Read the model definition and answer for the solid it produces. Units are mm, in the model's axes. A direction names the side the tool comes from. Coordinates: 2 decimals unless noted, no trailing zeros. Order: outer loops, then holes, each group sorted by start corner. A loop starts at its lowest first (then second) coordinate and runs counter-clockwise, first axis right, second up. Notation, with made-up numbers: M 22.5,85 L 71.5,85 A27 cw 71.5,105 Z; hole C 11.25,52 d6. An arc over 180 degrees is marked long. Use a Markdown table: item, result. Add a question column.
1) Each of these flat-tipped pins is pushed along its axis until it touches: pin 1 Ø2 at (x, y) = (45.5, -19) entering from -Z; pin 2 Ø8 at (y, z) = (-32, 12) entering from +X; pin 3 Ø5.5 at (x, y) = (402.5, -28) entering from -Z; pin 4 Ø10 at (x, z) = (143.5, 24) entering from +Y. Where does it stop, or does it pass through?
2) For faces 5 (the face through (395, -25, 11.195)), 6 (the face through (200, -29, 19.35)), 7 (the face through (431, -34, 12)), determine the directions among +Z, -Z, +X, -X, +Y, -Y from which every point of the face is accessible in a straight line to the end or side of a thin tool.
3) The mould has two halves that part along X. Classify faces 1 (the face through (385, -25, 6)), 2 (the face through (498, -10, 17)), 3 (the face through (75, -25, 0)), 4 (the face through (87, -31, 13)): released by +X, released by -X, zero draft, split by the parting line, or undercut.
4) Find the intervals of material crossed by probe 1 along Y at (x, z) = (402.5, 20.25); probe 2 along X at (y, z) = (-15.5, 8.5); probe 3 along X at (y, z) = (-21, 22), in increasing order. Write a range as [from, to].
5) Find section A-A on x = 194. Write down the section's boundary in (y, z).
from build123d import *

# Parameters (mm, degrees)
SKETCH6_R             = 9
BOSS_EXTRUDE2_DEPTH   = 27
CHAMFER1_SIZE         = 4
CUT_EXTRUDE5_DEPTH    = 28
CHAMFER2_SIZE         = 0.5
CHAMFER3_SIZE         = 0.5
SKETCH8_W             = 30
SKETCH8_H             = 16
CUT_EXTRUDE6_DEPTH    = 27
SKETCH8_3_W           = 30
SKETCH8_3_H           = 27
CUT_EXTRUDE7_DEPTH    = 4
FILLET1_R             = 2
CUT_EXTRUDE8_DEPTH    = 1
SKETCH11_W            = 21
SKETCH11_H            = 28.648086621
CUT_EXTRUDE9_DEPTH    = 51
SKETCH12_W            = 21
SKETCH12_H            = 8
CUT_EXTRUDE10_DEPTH   = 20
SKETCH13_W            = 21
SKETCH13_H            = 30.21821637
CUT_EXTRUDE11_DEPTH   = 51
CUT_EXTRUDE12_DEPTH   = 34.38478555
SKETCH15_R            = 1.75
CUT_EXTRUDE13_DEPTH   = 28
SKETCH16_R            = 3.25
CUT_EXTRUDE14_DEPTH   = 3.5
FILLET2_R             = 1
M4_TAPPED_HOLE1_D     = 3.3
M4_TAPPED_HOLE1_DEPTH = 8
M4_TAPPED_HOLE1_TIP   = 0.991420021
M3_TAPPED_HOLE1_D     = 2.5
M3_TAPPED_HOLE1_DEPTH = 6
M3_TAPPED_HOLE1_TIP   = 0.751075774
M3_TAPPED_HOLE2_D     = 2.5
M3_TAPPED_HOLE2_DEPTH = 6
M3_TAPPED_HOLE2_TIP   = 0.751075774
M3_TAPPED_HOLE3_D     = 2.5
M3_TAPPED_HOLE3_DEPTH = 6
M3_TAPPED_HOLE3_TIP   = 0.751075774
M3_TAPPED_HOLE4_D     = 2.5
M3_TAPPED_HOLE4_DEPTH = 6
M3_TAPPED_HOLE4_TIP   = 0.751075774
M3_TAPPED_HOLE5_D     = 2.5
M3_TAPPED_HOLE5_DEPTH = 6
M3_TAPPED_HOLE5_TIP   = 0.751075774
SKETCH29_W            = 25.5
SKETCH29_H            = 8
CUT_EXTRUDE15_DEPTH   = 17.61521445


with BuildPart() as part:
    # Sketch6 → Boss-Extrude2 (new body)
    with BuildSketch(Plane.XY):
        Polygon((112, -50), (477, -50), (477, -19), (498, -19), (498, 0), (214.9, 0), (214.9, -16.61521445), (137.1, -16.61521445), (137.1, 0), (0, 0), (0, -50), (87, -50), (87, -16.61521445), (112, -16.61521445), align=None)
        with Locations((27, -37)):
            Circle(SKETCH6_R, mode=Mode.SUBTRACT)
        with Locations((461, -37)):
            Circle(SKETCH6_R, mode=Mode.SUBTRACT)
    extrude(amount=BOSS_EXTRUDE2_DEPTH)

    # Chamfer1
    chamfer1_edges = [part.edges().sort_by_distance(p)[0] for p in [
        (0, -50, 13.5),
    ]]
    chamfer(chamfer1_edges, length=CHAMFER1_SIZE)

    # Sketch7 → Cut-Extrude5 (cut, through all)
    with BuildSketch(Plane.XY.offset(27)):
        with BuildLine():
            Line((151, -41.853199992), (151, -50))
            Line((151, -50), (165, -50))
            Line((165, -50), (165, -41.853199992))
            ThreePointArc((165, -41.853199992), (158, -34.853199992), (151, -41.853199992))
        make_face()
        with BuildLine():
            Line((187, -50), (201, -50))
            Line((201, -50), (201, -41.853199992))
            ThreePointArc((201, -41.853199992), (194, -34.853199992), (187, -41.853199992))
            Line((187, -41.853199992), (187, -50))
        make_face()
    extrude(amount=-CUT_EXTRUDE5_DEPTH, mode=Mode.SUBTRACT)

    # Chamfer2
    chamfer2_edges = [part.edges().sort_by_distance(p)[0] for p in [
        (137.1, 0, 13.5),
        (214.9, 0, 13.5),
    ]]
    chamfer(chamfer2_edges, length=CHAMFER2_SIZE)

    # Chamfer3
    chamfer3_edges = [part.edges().sort_by_distance(p)[0] for p in [
        (0, 0, 13.5),
        (498, 0, 13.5),
        (477, -50, 13.5),
        (112, -50, 13.5),
        (87, -50, 13.5),
    ]]
    chamfer(chamfer3_edges, length=CHAMFER3_SIZE)

    # Sketch8 → Cut-Extrude6 (cut)
    with BuildSketch(Plane.XY.offset(27)):
        with Locations((431, -42)):
            Rectangle(SKETCH8_W, SKETCH8_H)
    extrude(amount=-CUT_EXTRUDE6_DEPTH, mode=Mode.SUBTRACT)

    # Sketch8<3> → Cut-Extrude7 (cut)
    with BuildSketch(Plane.XY.offset(27)):
        with Locations((431, -20.5)):
            Rectangle(SKETCH8_3_W, SKETCH8_3_H)
    extrude(amount=-CUT_EXTRUDE7_DEPTH, mode=Mode.SUBTRACT)

    # Fillet1
    fillet1_edges = [part.edges().sort_by_distance(p)[0] for p in [
        (416, -7, 25),
        (446, -7, 25),
    ]]
    fillet(fillet1_edges, radius=FILLET1_R)

    # Sketch10 → Cut-Extrude8 (cut)
    with BuildSketch(Plane.XY.offset(27)):
        Polygon((5, -4.129705764), (132.1, -4.129705764), (137.1, -5.469451726), (137.1, -4.129705764), (493, -4.129705764), (498, -5.469451726), (498.112682479, -4.129705764), (498.112682479, 0), (0, 0), (0, -4.129705764), (0, -5.469451726), align=None)
    extrude(amount=-CUT_EXTRUDE8_DEPTH, mode=Mode.SUBTRACT)

    # Sketch11 → Cut-Extrude9 (cut, through all)
    with BuildSketch(Plane.XZ.offset(50)):
        with Locations((53.5, -6.324043311)):
            Rectangle(SKETCH11_W, SKETCH11_H)
    extrude(amount=-CUT_EXTRUDE9_DEPTH, mode=Mode.SUBTRACT)

    # Sketch12 → Cut-Extrude10 (cut, through all)
    with BuildSketch(Plane.XZ.offset(19)):
        with Locations((487.5, 4)):
            Rectangle(SKETCH12_W, SKETCH12_H)
    extrude(amount=-CUT_EXTRUDE10_DEPTH, mode=Mode.SUBTRACT)

    # Sketch13 → Cut-Extrude11 (cut, through all)
    with BuildSketch(Plane.XZ.offset(50)):
        with Locations((395.5, -3.9138874)):
            Rectangle(SKETCH13_W, SKETCH13_H)
    extrude(amount=-CUT_EXTRUDE11_DEPTH, mode=Mode.SUBTRACT)

    # Sketch14 → Cut-Extrude12 (cut, through all)
    with BuildSketch(Plane(origin=(0, -16.61521445, 0), x_dir=(1, 0, 0), z_dir=(0, 1, 0))):
        Polygon((137.1, -27), (214.9, -27), (214.9, -19.35), (184, -19.35), (184, -16.3), (167.5, -16.3), (167.5, -19.35), (137.1, -19.35), align=None)
    extrude(amount=-CUT_EXTRUDE12_DEPTH, mode=Mode.SUBTRACT)

    # Sketch15 → Cut-Extrude13 (cut, through all)
    with BuildSketch(Plane.XY.offset(27)):
        with Locations((45.5, -19)):
            Circle(SKETCH15_R)
        with Locations((60.5, -19)):
            Circle(SKETCH15_R)
        with Locations((45.5, -28)):
            Circle(SKETCH15_R)
        with Locations((60.5, -28)):
            Circle(SKETCH15_R)
        with Locations((387.5, -19)):
            Circle(SKETCH15_R)
        with Locations((402.5, -19)):
            Circle(SKETCH15_R)
        with Locations((387.5, -28)):
            Circle(SKETCH15_R)
        with Locations((402.5, -28)):
            Circle(SKETCH15_R)
    extrude(amount=-CUT_EXTRUDE13_DEPTH, mode=Mode.SUBTRACT)

    # Sketch16 → Cut-Extrude14 (cut)
    with BuildSketch(Plane.XY.offset(27)):
        with Locations((45.5, -19)):
            Circle(SKETCH16_R)
        with Locations((60.5, -19)):
            Circle(SKETCH16_R)
        with Locations((60.5, -28)):
            Circle(SKETCH16_R)
        with Locations((45.5, -28)):
            Circle(SKETCH16_R)
        with Locations((387.5, -19)):
            Circle(SKETCH16_R)
        with Locations((402.5, -19)):
            Circle(SKETCH16_R)
        with Locations((402.5, -28)):
            Circle(SKETCH16_R)
        with Locations((387.5, -28)):
            Circle(SKETCH16_R)
    extrude(amount=-CUT_EXTRUDE14_DEPTH, mode=Mode.SUBTRACT)

    # Fillet2
    fillet2_edges = [part.edges().sort_by_distance(p)[0] for p in [
        (137.1, -16.61521445, 9.675),
        (214.9, -16.61521445, 9.675),
    ]]
    fillet(fillet2_edges, radius=FILLET2_R)

    # M4 Tapped Hole1
    with Locations(Plane.XY.offset(19.35)):
        with Locations((146, -27), (206, -27)):
            Hole(M4_TAPPED_HOLE1_D / 2, depth=M4_TAPPED_HOLE1_DEPTH)
            with Locations((0, 0, -(M4_TAPPED_HOLE1_DEPTH + M4_TAPPED_HOLE1_TIP / 2))):  # 118° drill point
                Cone(0, M4_TAPPED_HOLE1_D / 2, M4_TAPPED_HOLE1_TIP, mode=Mode.SUBTRACT)

    # M3 Tapped Hole1
    with Locations(Plane.XY.offset(27)):
        with Locations((13, -10), (33, -10), (80, -10), (110, -10), (251, -10), (303, -10), (373, -10), (358, -10)):
            Hole(M3_TAPPED_HOLE1_D / 2, depth=M3_TAPPED_HOLE1_DEPTH)
            with Locations((0, 0, -(M3_TAPPED_HOLE1_DEPTH + M3_TAPPED_HOLE1_TIP / 2))):  # 118° drill point
                Cone(0, M3_TAPPED_HOLE1_D / 2, M3_TAPPED_HOLE1_TIP, mode=Mode.SUBTRACT)

    # M3 Tapped Hole2
    with Locations(Plane(origin=(0, -19, 0), x_dir=(-1, 0, 0), z_dir=(0, -1, 0))):
        with Locations((-486, -12), (-494, -12)):
            Hole(M3_TAPPED_HOLE2_D / 2, depth=M3_TAPPED_HOLE2_DEPTH)
            with Locations((0, 0, -(M3_TAPPED_HOLE2_DEPTH + M3_TAPPED_HOLE2_TIP / 2))):  # 118° drill point
                Cone(0, M3_TAPPED_HOLE2_D / 2, M3_TAPPED_HOLE2_TIP, mode=Mode.SUBTRACT)

    # M3 Tapped Hole3
    with Locations(Plane(origin=(0, -34, 0), x_dir=(-1, 0, 0), z_dir=(0, -1, 0))):
        with Locations((-424.5, -15.24), (-437.5, -15.24)):
            Hole(M3_TAPPED_HOLE3_D / 2, depth=M3_TAPPED_HOLE3_DEPTH)
            with Locations((0, 0, -(M3_TAPPED_HOLE3_DEPTH + M3_TAPPED_HOLE3_TIP / 2))):  # 118° drill point
                Cone(0, M3_TAPPED_HOLE3_D / 2, M3_TAPPED_HOLE3_TIP, mode=Mode.SUBTRACT)

    # M3 Tapped Hole4
    with Locations(Plane(origin=(0, -50, 0), x_dir=(-1, 0, 0), z_dir=(0, -1, 0))):
        with Locations((-138.7, -12.9), (-146.7, -12.9)):
            Hole(M3_TAPPED_HOLE4_D / 2, depth=M3_TAPPED_HOLE4_DEPTH)
            with Locations((0, 0, -(M3_TAPPED_HOLE4_DEPTH + M3_TAPPED_HOLE4_TIP / 2))):  # 118° drill point
                Cone(0, M3_TAPPED_HOLE4_D / 2, M3_TAPPED_HOLE4_TIP, mode=Mode.SUBTRACT)

    # M3 Tapped Hole5
    with Locations(Plane(origin=(0, -16.61521445, 0), x_dir=(-1, 0, 0), z_dir=(0, -1, 0))):
        with Locations((-95.5, -12), (-103.5, -12)):
            Hole(M3_TAPPED_HOLE5_D / 2, depth=M3_TAPPED_HOLE5_DEPTH)
            with Locations((0, 0, -(M3_TAPPED_HOLE5_DEPTH + M3_TAPPED_HOLE5_TIP / 2))):  # 118° drill point
                Cone(0, M3_TAPPED_HOLE5_D / 2, M3_TAPPED_HOLE5_TIP, mode=Mode.SUBTRACT)

    # Sketch29 → Cut-Extrude15 (cut, through all)
    with BuildSketch(Plane.XZ.offset(16.61521445)):
        with Locations((99.75, 4)):
            Rectangle(SKETCH29_W, SKETCH29_H)
    extrude(amount=-CUT_EXTRUDE15_DEPTH, mode=Mode.SUBTRACT)


solid = part.part
Check result:
| question | item | result |
|---|---|---|
| 1 | pin 1 | passes through |
| 1 | pin 2 | stops at x = 477 |
| 1 | pin 3 | stops at z = 11.2 |
| 1 | pin 4 | stops at y = -16.62 |
| 2 | face 5 | -Z, +Y, -Y |
| 2 | face 6 | +Z, +Y, -Y |
| 2 | face 7 | +Z, -Z, -Y |
| 3 | face 1 | undercut |
| 3 | face 2 | released by +X |
| 3 | face 3 | zero draft |
| 3 | face 4 | undercut |
| 4 | probe 1 | y = [-50, -29.75], [-26.25, -20.75], [-17.25, 0] |
| 4 | probe 2 | x = [0, 137.1], [214.9, 385], [406, 498] |
| 4 | probe 3 | x = [0, 87], [112, 137.1], [214.9, 477] |
| 5 | outline | M -34.85,0 L -16.62,0 L -16.62,19.35 L -34.85,19.35 Z |
